from build123d import *

# Parameters (mm, degrees)
SKETCH_1_R               = 16
SKETCH_1_R_2             = 15
EXTRUDE_1_DEPTH          = 4
SKETCH_2_R               = 0.75
CUT_EXTRUDE_1_DEPTH      = 17
PATTERN_CIRCULAR_1_COUNT = 16
SKETCH_3_W               = 36.79853237
SKETCH_3_H               = 11.94610836
CUT_EXTRUDE_2_DEPTH      = 17.0000001


with BuildPart() as part:
    # ｽｹｯﾁ1 → ﾎﾞｽ - 押し出し1 (new body)
    with BuildSketch(Plane.XY):
        Circle(SKETCH_1_R)
        Circle(SKETCH_1_R_2, mode=Mode.SUBTRACT)
    extrude(amount=EXTRUDE_1_DEPTH)

    # ｽｹｯﾁ2 → ｶｯﾄ - 押し出し1 (cut, through all)
    with BuildSketch(Plane(origin=(0, 0, 0), x_dir=(1, 0, 0), z_dir=(0, 1, 0))):
        with Locations((0, -1.957637914)):
            Circle(SKETCH_2_R)
    cut_extrude_1 = extrude(amount=-CUT_EXTRUDE_1_DEPTH, mode=Mode.SUBTRACT)

    # 円形ﾊﾟﾀｰﾝ1: ｶｯﾄ - 押し出し1 ×16 about axis
    pattern_circular_1_axis = Axis((0, 0, 0), (0, 0, 1))
    for i in range(1, PATTERN_CIRCULAR_1_COUNT):
        add(cut_extrude_1.rotate(pattern_circular_1_axis, i * 360 / PATTERN_CIRCULAR_1_COUNT), mode=Mode.SUBTRACT)

    # ｽｹｯﾁ3 → ｶｯﾄ - 押し出し2 (cut, through all)
    with BuildSketch(Plane(origin=(0, 0, 0), x_dir=(1, 0, 0), z_dir=(0, 1, 0))):
        with Locations((0, -2.028241391)):
            Rectangle(SKETCH_3_W, SKETCH_3_H)
    extrude(amount=-CUT_EXTRUDE_2_DEPTH, mode=Mode.SUBTRACT)


solid = part.part
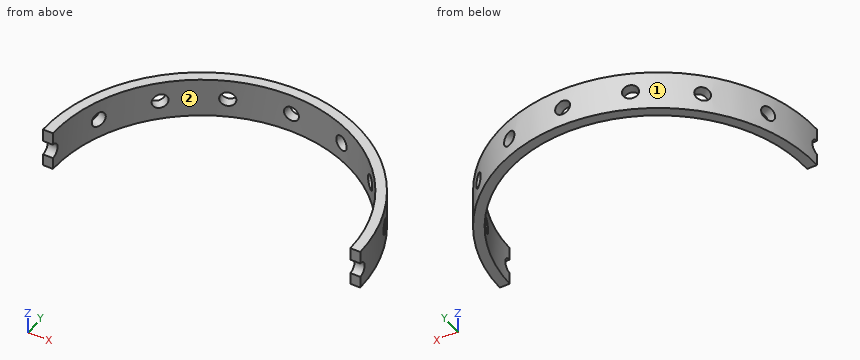
For this review, take the finished solid that the model builds, in its own axes (mm). Face numbers are marked on the shaded views. Round coordinates to 2 decimals unless told otherwise and drop trailing zeros. Loops run counter-clockwise (first coordinate to the right, second up) from the corner with the lowest first, then second, coordinate; pieces in that order, holes last. Notation, with made-up numbers: (67.5, 8) - (86.5, 8) arc R29 ccw to (86.5, 30) - close; hole circle Ø4 at (-29.75, 45.5). An arc over 180 degrees is marked (long way). Use one line per item in the form item = value.
Item 1: Consider section B-B on y = 2. Write out the cut boundary in (x, z).
Answers:
outline = (-15.87, 0) - (-14.87, 0) - (-14.87, 4) - (-15.87, 4) - close; (14.87, 0) - (15.87, 0) - (15.87, 4) - (14.87, 4) - close
Item 2: Consider section A-A on x = 0. Write out the cut boundary in (y, z).
Answers:
outline = (15, 0) - (16, 0) - (16, 1.21) - (15, 1.21) - close; (15, 2.71) - (16, 2.71) - (16, 4) - (15, 4) - close
Item 3: Consider section D-D on x = 3.5. Write out the cut boundary in (y, z).
Answers:
outline = (14.59, 0) - (15.61, 0) - (15.61, 4) - (14.59, 4) - close
Item 4: For line 1 (Z direction, x = 0, y = 15.75); line 2 (X direction, y = 3, z = 0.4); line 3 (X direction, y = 12.5, z = 3.5), list the stretches that pass through material, from the lowest coordinate up.
Answers:
line_1 = 0 to 1.21, 2.71 to 4
line_2 = -15.72 to -14.7, 14.7 to 15.72
line_3 = -9.99 to -8.29, 8.29 to 9.99
Item 5: Mouldability with a two-part tool opening along X and no side actions: class the marked faces 1 and 2 as +X half, -X half, draft (parallel to the pull), parting line (faces both ways), or undercut.
Answers:
face_1 = parting line
face_2 = undercut
Item 6: Clearance check with flat-ended pins moving along their axes: P1, Ø8, axis at x = 0, y = 10, coming from the +Z side; P2, Ø2, axis at x = 12.5, z = 1.5, coming from the -Y side; P3, Ø2, axis at x = -9, z = 1, coming from the +Y side. State where each tip first meets the part, or that it passes through.
Answers:
P1 = through
P2 = 6.54
P3 = 13.86
Item 7: Consider section C-C on z = 3.05. Write out the cut boundary in (x, y), then the cut area to 3 significant figures.
Answers:
outline = (-16, 0) - (-15, 0) arc R15 cw to (15, 0) - (16, 0) arc R16 ccw to start
area = 48.7 mm^2
